Autodesk Inventor part; units mm, degrees
ref_plane "YZ Plane" through (0, 0, 0) normal (1, 0, 0) x (0, 1, 0)
ref_plane "XZ Plane" through (0, 0, 0) normal (0, 1, 0) x (-1, 0, 0)
ref_plane "XY Plane" through (0, 0, 0) normal (0, 0, 1) x (1, 0, 0)
sketch "Boceto3" plane through (0, 0, 0) normal (0, 0, 1) x (1, 0, 0)
  line L0 (1, 1.5) -> (16, 1.5)
  line L1 (16, 1.5) -> (16, -1.5)
  line L2 (16, -1.5) -> (1, -1.5)
  line L3 (1, -1.5) -> (1, 1.5)
  point P0 (0, 0)
  point P1 (1, 0)
  dimension "d4" = 3
  dimension "d5" = 15
  dimension "d6" = 16
coil "Bobina1" sketch "Boceto3" operation add axis through (0, -10, 0) along (0, -1, 0) pitch 16 turns 3.5 hand right
properties part number "bobina"
Here's how the part is built. I have some questions about the finished solid (model axes, mm). A direction names the side the tool comes from. Coordinates: 2 decimals unless noted, no trailing zeros. Use a Markdown table: item, result. Add a question column.
(1) If we section it at A-A, the plane z = 9.5: State how many separate pieces and enclosed holes the cut face has, and give its area (3 significant figures).
(2) For faces 1 (the flat face through (8, 0, 0)), 2 (the flat face through (-8, -56, 0)), which set-ups out of +Z, -Z, +X, -X, +Y, -Y let a thin tool reach every point of the face, with its end or its side?
(3) Please list where these lines run through material, in increasing order: line 1 (Y direction, x = 1, z = -6.5); line 2 (Y direction, x = 4.5, z = -10); line 3 (Y direction, x = -12, z = 7).
(4) I'm going to push flat-ended pins straight in: P1, Ø12, axis at x = 12, z = 7, coming from the -Y side; P2, Ø12, axis at x = 12.5, y = -51, coming from the +Z side; P3, Ø3.5, axis at x = -10.5, y = -56, coming from the -Z side. Where does each tip first touch, or does it pass through?
Outcome:
| question | item | result |
|---|---|---|
| 1 | separate pieces | 4 |
| 1 | enclosed holes | 0 |
| 1 | area | 309 mm^2 |
| 2 | face 1 | -Z, +X, -X, +Y |
| 2 | face 2 | -Z, +X, -X, -Y |
| 3 | line 1 | y = -45.89 to -42.89, -29.89 to -26.89, -13.89 to -10.89 |
| 3 | line 2 | y = -46.58 to -43.58, -30.58 to -27.58, -14.58 to -11.58 |
| 3 | line 3 | y = -56.16 to -53.16, -40.16 to -37.16, -24.16 to -21.16, -8.16 to -5.16 |
| 4 | P1 | stops at y = -51.98 |
| 4 | P2 | stops at z = 14.62 |
| 4 | P3 | stops at z = 0 |
